The model under review builds one solid part; all positions refer to its coordinate system, in mm. A direction names the side the tool comes from. Coordinates: 2 decimals unless noted, no trailing zeros. Write each loop counter-clockwise with the first axis right and the second up, starting at its lowest first coordinate (ties: lowest second). Pieces come first, ordered by that corner, then holes.
```python
from build123d import *

# Parameters (mm, degrees)
SKETCH1_W           = 40
SKETCH1_H           = 20
BOSS_EXTRUDE1_DEPTH = 2.9718
BOSS_EXTRUDE2_DEPTH = 2.9718
SKETCH3_W           = 3.302
SKETCH3_H           = 20
CUT_EXTRUDE1_DEPTH  = 3.9718
SKETCH4_W           = 10
SKETCH4_H           = 3.81
BOSS_EXTRUDE3_DEPTH = 2.9718


with BuildPart() as part:
    # Sketch1 → Boss-Extrude1 (new body)
    with BuildSketch(Plane.XY):
        Rectangle(SKETCH1_W, SKETCH1_H)
    extrude(amount=BOSS_EXTRUDE1_DEPTH)

    # Sketch2 → Boss-Extrude2 (add)
    with BuildSketch(Plane.XY.offset(2.9718)):
        Polygon((-20, 10), (-30, -10), (-20, -10), align=None)
        Polygon((20, -10), (20, 10), (30, -10), align=None)
    extrude(amount=-BOSS_EXTRUDE2_DEPTH)

    # Sketch3 → Cut-Extrude1 (cut, through all)
    with BuildSketch(Plane.XY.offset(2.9718)):
        with Locations((-11.651, 10)):
            Rectangle(SKETCH3_W, SKETCH3_H)
        with Locations((11.651, 10)):
            Rectangle(SKETCH3_W, SKETCH3_H)
    extrude(amount=-CUT_EXTRUDE1_DEPTH, mode=Mode.SUBTRACT)

    # Sketch4 → Boss-Extrude3 (add)
    with BuildSketch(Plane.XY.offset(2.9718)):
        with Locations((-15, -11.905)):
            Rectangle(SKETCH4_W, SKETCH4_H)
        with Locations((15, -11.905)):
            Rectangle(SKETCH4_W, SKETCH4_H)
    extrude(amount=-BOSS_EXTRUDE3_DEPTH)


solid = part.part
```
Item 1: To check wall thickness, follow line 1 along X through (y, z) = (-10.25, 1.7); line 2 along X through (y, z) = (7.75, 1.05) (3 decimals); line 3 along X through (y, z) = (3.25, 1.6) (3 decimals). State the ranges of each line that lie inside material, in increasing order.
Solved:
line 1: x = -20 to -10, 10 to 20
line 2: x = -21.125 to -13.302, -10 to 10, 13.302 to 21.125
line 3: x = -23.375 to -13.302, -10 to 10, 13.302 to 23.375
Item 2: Take a section at C-C, the plane z = 1.15. Write out the cut boundary in (x, y).
Solved:
outline: (-30, -10) - (-20, -10) - (-20, -13.81) - (-10, -13.81) - (-10, -10) - (10, -10) - (10, -13.81) - (20, -13.81) - (20, -10) - (30, -10) - (20, 10) - (13.3, 10) - (13.3, 0) - (10, 0) - (10, 10) - (-10, 10) - (-10, 0) - (-13.3, 0) - (-13.3, 10) - (-20, 10) - close
Item 3: Mouldability with a two-part tool opening along X and no side actions: class faces 1 (the face through (-13.302, 5, 2)), 2 (the face through (-20, -12, 2)), 3 (the face through (-17, 10, 1)) as pulls with the +X half, pulls with the -X half, needs draft (parallel to the pull), parting line crosses it, or undercut.
Solved:
face 1: undercut
face 2: pulls with the -X half
face 3: needs draft
Item 4: Take a section at D-D, the plane x = -5. Write out the cut boundary in (y, z).
Solved:
outline: (-10, 0) - (10, 0) - (10, 2.97) - (-10, 2.97) - close
Item 5: Take a section at A-A, the plane y = 3.5. Write out the cut boundary in (x, z), plus the area to 3 significant figures.
Solved:
outline: (-23.25, 0) - (-13.3, 0) - (-13.3, 2.97) - (-23.25, 2.97) - close; (-10, 0) - (10, 0) - (10, 2.97) - (-10, 2.97) - close; (13.3, 0) - (23.25, 0) - (23.25, 2.97) - (13.3, 2.97) - close
area: 119 mm2
Item 6: For pin 1 (8 mm diameter, centred on x = -23, y = 4.5, fed in from -Z); pin 2 (1.5 mm diameter, centred on x = 26, z = 1.5, fed in from -Y); pin 3 (0.9 mm diameter, centred on y = -12, z = 1, fed in from -X); pin 4 (1.5 mm diameter, centred on y = 7, z = 1, fed in from -X) (3 decimals), all flat-tipped, find the tip position at first contact; note any pin that passes through.
Solved:
pin 1: stops at z = 0
pin 2: stops at y = -10
pin 3: stops at x = -20
pin 4: stops at x = -21.875
Item 7: Machinability: for faces 4 (the face through (-25, -10, 2)), 5 (the face through (25, -10, 2)), 6 (the face through (10, -12, 2)), 7 (the face through (-12, 0, 2)), which of the approach directions +Z, -Z, +X, -X, +Y, -Y give a long, thin tool a straight path to every point of the face, cutting with its end or side? Answer none if there is none.
Solved:
face 4: +Z, -Z, -X, -Y
face 5: +Z, -Z, +X, -Y
face 6: +Z, -Z, -Y
face 7: +Z, -Z, +Y
Item 8: Take a section at B-B, the plane y = -12. Write out the cut boundary in (x, z), plus the area to 3 significant figures.
Solved:
outline: (-20, 0) - (-10, 0) - (-10, 2.97) - (-20, 2.97) - close; (10, 0) - (20, 0) - (20, 2.97) - (10, 2.97) - close
area: 59.4 mm2
